Autodesk Inventor part; units mm, degrees
ref_plane "YZ Plane" through (0, 0, 0) normal (1, 0, 0) x (0, 1, 0)
ref_plane "XZ Plane" through (0, 0, 0) normal (0, 1, 0) x (-1, 0, 0)
ref_plane "XY Plane" through (0, 0, 0) normal (0, 0, 1) x (1, 0, 0)
sketch "スケッチ1" plane through (0, 0, 0) normal (0, 0, 1) x (1, 0, 0)
  circle A0 centre (0, 0) radius 9
  dimension "d0" = 18
extrude "押し出し1" add sketch "スケッチ1" along normal blind 2
sketch "スケッチ2" plane through (0, 0, 2) normal (0, 0, 1) x (1, 0, 0)
  line L0 (0, 7.2169) -> (6.25, 3.6084)
  line L1 (6.25, 3.6084) -> (6.25, -3.6084)
  line L2 (6.25, -3.6084) -> (0, -7.2169)
  line L3 (0, -7.2169) -> (-6.25, -3.6084)
  line L4 (-6.25, -3.6084) -> (-6.25, 3.6084)
  line L5 (-6.25, 3.6084) -> (0, 7.2169)
  point P0 (0, 0)
  point P1 (0, 0)
  dimension "d3" = 12.5
extrude "押し出し2" add sketch "スケッチ2" along normal blind 7
sketch "スケッチ3" plane through (0, 0, 9) normal (0, 0, 1) x (1, 0, 0)
  circle A0 centre (0, 0) radius 6.25
  dimension "d6" = 12.5
extrude "押し出し3" add sketch "スケッチ3" along normal blind 2
sketch "スケッチ4" plane through (0, 0, 11) normal (0, 0, 1) x (1, 0, 0)
  point P0 (0, 0)
hole "穴1" at (0, 0, 11) direction (0, 0, -1) diameter 6.647 end through all
chamfer "面取り1" distance 0.5 angle 45 2 edges at (0, 3.3235, 11) (0, 3.3235, 0)
chamfer "面取り2" distance 1.5 angle 45 1 edges at (-9, 0, 2)
properties part number "nut" material "アルミニウム 6061"
For this review, take the finished solid that the model builds, in its own axes (mm). A direction names the side the tool comes from. Give positions to 0.01 mm unless a question says otherwise; leave off trailing zeros. Order: outer loops, then holes, each group sorted by start corner. A loop starts at its lowest first (then second) coordinate and runs counter-clockwise, first axis right, second up. Notation, with made-up numbers: (27.5, 82) -> (67.5, 82) arc R27 cw to (67.5, 101) -> close; hole circle Ø10 at (-27, -12). An arc over 180 degrees is marked (long way). Write item = value, one per line.
1) Insertion check: pin 1 (4 mm diameter, centred on x = -6, z = 4, fed in from +Y); pin 2 (2 mm diameter, centred on y = -1.5, z = 5, fed in from +X); pin 3 (1.5 mm diameter, centred on x = 1.5, z = 4, fed in from -Y). Each pin has a flat end and moves straight along its axis. Give the tip position at first contact, or say it passes through.
Findings:
pin_1 = 4.91
pin_2 = 6.25
pin_3 = -6.78
2) To check wall thickness, follow L1, parallel to X at y = 0, z = 7.25; L2, parallel to Z at x = -6, y = -4.5; L3, parallel to X at y = -1, z = 6.75. State the ranges of each line that lie inside material, in increasing order. Write a range as from..to.
Findings:
L1 = -6.25..-3.32, 3.32..6.25
L2 = 0..2
L3 = -6.25..-3.17, 3.17..6.25
3) We need section A-A, the plane z = 8. Give the boundary of the cut face in (x, y).
Findings:
outline = (-6.25, -3.61) -> (0, -7.22) -> (6.25, -3.61) -> (6.25, 3.61) -> (0, 7.22) -> (-6.25, 3.61) -> close; hole circle Ø6.65 at (0, 0)
4) Draft analysis for pull direction X (two halves, no side actions). For faces 6 (the face through (-1.172, -8.923, 0.246)), 7 (the face through (1.27, -3.07, 5.43)), 8 (the face through (-6, 3, 9)), state which applies: pulls with the +X half, pulls with the -X half, needs draft (parallel to the pull), parting line crosses it, or undercut.
Findings:
face_6 = parting line crosses it
face_7 = undercut
face_8 = needs draft
5) For faces 1 (the face through (-6, -3, 9)), 2 (the face through (6, 3, 9)), 3 (the face through (-6.25, 0, 5)), 4 (the face through (0, -6.4, 9)), 5 (the face through (3, 6, 2)), list the 3-axis set-ups (+Z, -Z, +X, -X, +Y, -Y) from which the entire face can be reached by the end or side of a thin tool; tool diameter is ignored.
Findings:
face_1 = +Z, -X, -Y
face_2 = +Z, +X, +Y
face_3 = +Z, -X, +Y, -Y
face_4 = +Z, -Y
face_5 = +Z
